Here's how the part is built. I have some questions about the finished solid (model axes, mm). Round coordinates to 2 decimals unless told otherwise and drop trailing zeros. Loops run counter-clockwise (first coordinate to the right, second up) from the corner with the lowest first, then second, coordinate; pieces in that order, holes last. Notation, with made-up numbers: (51.5, 34.25) -> (89.5, 34.25) arc R14 cw to (89.5, 49.25) -> close; hole circle Ø5 at (17.5, 83.25). An arc over 180 degrees is marked (long way). Use CSV: the item, a comma, the result in double quotes. Start each with the question number.
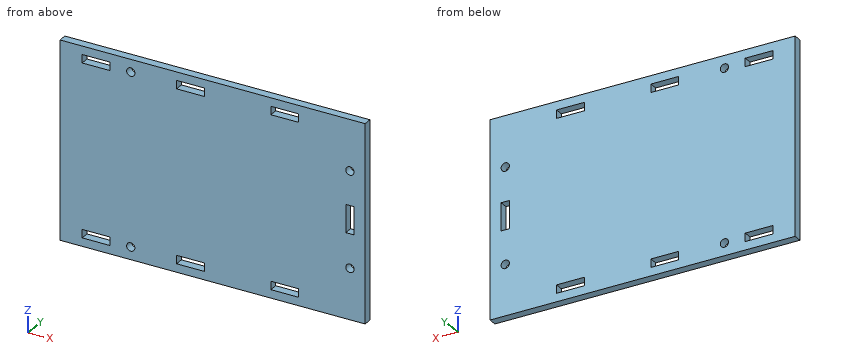
from build123d import *

# Parameters (mm, degrees)
SKETCH1_W           = 110
SKETCH1_H           = 71
SKETCH1_R           = 1.5
SKETCH1_W_2         = 10
SKETCH1_H_2         = 3
SKETCH1_W_3         = 3
SKETCH1_H_3         = 10
BOSS_EXTRUDE1_DEPTH = 3


with BuildPart() as part:
    # Sketch1 → Boss-Extrude1 (new body)
    with BuildSketch(Plane(origin=(0, 0, 0), x_dir=(1, 0, 0), z_dir=(0, 1, 0))):
        with Locations((-55, 35.5)):
            Rectangle(SKETCH1_W, SKETCH1_H)
        with Locations(Location((-5.5, 18.25, 0), (0, 0, 270))):
            Circle(SKETCH1_R, mode=Mode.SUBTRACT)
        with Locations(Location((-5.5, 52.75, 0), (0, 0, 90))):
            Circle(SKETCH1_R, mode=Mode.SUBTRACT)
        with Locations(Location((-84.5, 4.5, 0), (0, 0, 270))):
            Circle(SKETCH1_R, mode=Mode.SUBTRACT)
        with Locations(Location((-84.5, 66.5, 0), (0, 0, 90))):
            Circle(SKETCH1_R, mode=Mode.SUBTRACT)
        with Locations((-63, 4.5)):
            Rectangle(SKETCH1_W_2, SKETCH1_H_2, mode=Mode.SUBTRACT)
        with Locations((-5.5, 35.5)):
            Rectangle(SKETCH1_W_3, SKETCH1_H_3, mode=Mode.SUBTRACT)
        with Locations((-29, 4.5)):
            Rectangle(SKETCH1_W_2, SKETCH1_H_2, mode=Mode.SUBTRACT)
        with Locations((-97, 4.5)):
            Rectangle(SKETCH1_W_2, SKETCH1_H_2, mode=Mode.SUBTRACT)
        with Locations((-29, 66.5)):
            Rectangle(SKETCH1_W_2, SKETCH1_H_2, mode=Mode.SUBTRACT)
        with Locations((-63, 66.5)):
            Rectangle(SKETCH1_W_2, SKETCH1_H_2, mode=Mode.SUBTRACT)
        with Locations((-97, 66.5)):
            Rectangle(SKETCH1_W_2, SKETCH1_H_2, mode=Mode.SUBTRACT)
    extrude(amount=BOSS_EXTRUDE1_DEPTH)


solid = part.part
Q1. Will this pin go through, and if not, where does the flat tip stop? pin 1 Ø2.5 at (x, z) = (-5.5, -18.25) entering from +Y.
Q2. I want a section at B-B, the plane z = -33.5. List the corners of the cut face in (x, y) for me.
Q3. I want a section at D-D, the plane z = -4.5. List the corners of the cut face in (x, y) for me, then the cut area to 3 significant figures.
Q4. I want a section at A-A, the plane x = -29. List the corners of the cut face in (y, z) for me.
Q5. I need wall thicknesses on line 1 along Z through (x, y) = (-84.5, 0.7); line 2 along X through (y, z) = (1.8, -4.5); line 3 along X through (y, z) = (1.8, -18.25). Which ranges of each line are inside material? Lowest first, please.
Q6. I want a section at C-C, the plane x = -5.5. List the corners of the cut face in (y, z) for me.
Values found:
1,pin 1,"through"
2,outline,"(-110, 0) -> (-7, 0) -> (-7, 3) -> (-110, 3) -> close; (-4, 0) -> (0, 0) -> (0, 3) -> (-4, 3) -> close"
3,outline,"(-110, 0) -> (-102, 0) -> (-102, 3) -> (-110, 3) -> close; (-92, 0) -> (-86, 0) -> (-86, 3) -> (-92, 3) -> close; (-83, 0) -> (-68, 0) -> (-68, 3) -> (-83, 3) -> close; (-58, 0) -> (-34, 0) -> (-34, 3) -> (-58, 3) -> close; (-24, 0) -> (0, 0) -> (0, 3) -> (-24, 3) -> close"
3,area,"231 mm2"
4,outline,"(0, -71) -> (3, -71) -> (3, -68) -> (0, -68) -> close; (0, -65) -> (3, -65) -> (3, -6) -> (0, -6) -> close; (0, -3) -> (3, -3) -> (3, 0) -> (0, 0) -> close"
5,line 1,"-71 to -68, -65 to -6, -3 to 0"
5,line 2,"-110 to -102, -92 to -86, -83 to -68, -58 to -34, -24 to 0"
5,line 3,"-110 to -7, -4 to 0"
6,outline,"(0, -71) -> (3, -71) -> (3, -54.25) -> (0, -54.25) -> close; (0, -51.25) -> (3, -51.25) -> (3, -40.5) -> (0, -40.5) -> close; (0, -30.5) -> (3, -30.5) -> (3, -19.75) -> (0, -19.75) -> close; (0, -16.75) -> (3, -16.75) -> (3, 0) -> (0, 0) -> close"
